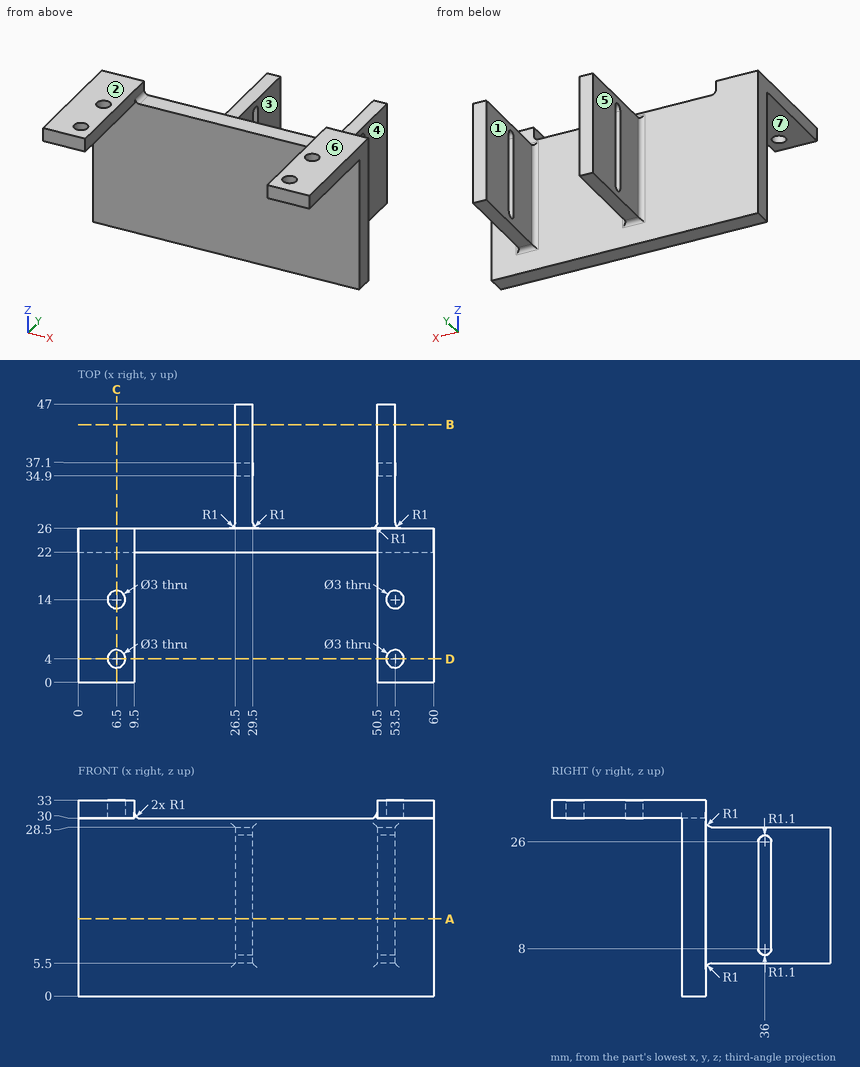
Geometry check sheet. Reference: drawing and pictorial views, mm from the part's lowest x, y, z. A direction names the side the tool comes from. Coordinates: 2 decimals unless noted, no trailing zeros. Order: outer loops, then holes, each group sorted by start corner. A loop starts at its lowest first (then second) coordinate and runs counter-clockwise, first axis right, second up. Notation, with made-up numbers: M 7.5,33 L 40.5,33 A19 cw 40.5,51 Z; hole C 56.5,84 d1. An arc over 180 degrees is marked long. Write each question's results on one line, items separated by ' | '. Start each with the question number.
1. Cross-section at A-A on z = 13. Record the cut outline in (x, y), and give its area (3 significant figures).
2. Cross-section at B-B on y = 43.5. Record the cut outline in (x, z).
3. Mould release check, pull along X, two halves, no side actions. Record for the marked faces 1, 2, 3 and 4: +X half, -X half, draft (parallel to the pull), parting line (faces both ways), or undercut.
4. Cross-section at C-C on x = 6.5. Record the cut outline in (y, z), and give its area (3 significant figures).
5. Access from +Z, -Z, +X, -X, +Y, -Y to the whole of each face (thin tool, end or side, straight path). Record for the marked faces 5, 6 and 7.
6. Cross-section at D-D on y = 4. Record the cut outline in (x, z), and give its area (3 significant figures).
7. Material ranges on probe 1 along Y at (x, z) = (53.5, 32.15); probe 2 along X at (y, z) = (45, 23); probe 3 along X at (y, z) = (19, 31), recorded low to high.
8. Go/stop test with flat-tipped pins: P1, Ø1.8, axis at x = 53.5, y = 4, coming from the +Z side; P2, Ø4, axis at x = 6.5, y = 14, coming from the -Z side; P3, Ø2, axis at x = 13, y = 23, coming from the +Z side; P4, Ø2.5, axis at x = 51.5, z = 16, coming from the -Y side. Record where each tip stops, or that it passes through.
Checks:
1) outline: M 0,22 L 60,22 L 60,26 L 54.5,26 A1 cw 53.5,27 L 53.5,34.9 L 50.5,34.9 L 50.5,27 A1 cw 49.5,26 L 30.5,26 A1 cw 29.5,27 L 29.5,34.9 L 26.5,34.9 L 26.5,27 A1 cw 25.5,26 L 0,26 Z; M 26.5,37.1 L 29.5,37.1 L 29.5,47 L 26.5,47 Z; M 50.5,37.1 L 53.5,37.1 L 53.5,47 L 50.5,47 Z | area: 354 mm²
2) outline: M 26.5,5.5 L 29.5,5.5 L 29.5,28.5 L 26.5,28.5 Z; M 50.5,5.5 L 53.5,5.5 L 53.5,28.5 L 50.5,28.5 Z
3) face 1: undercut | face 2: draft | face 3: undercut | face 4: +X half
4) outline: M 0,30 L 2.5,30 L 2.5,33 L 0,33 Z; M 5.5,30 L 12.5,30 L 12.5,33 L 5.5,33 Z; M 15.5,30 L 22,30 L 22,0 L 26,0 L 26,33 L 15.5,33 Z | area: 180 mm²
5) face 5: +Z, -Z, -X, +Y | face 6: +Z, +X, -X, +Y, -Y | face 7: -Z, +X, -X, -Y
6) outline: M 0,30 L 5,30 L 5,33 L 0,33 Z; M 8,30 L 9.5,30 L 9.5,33 L 8,33 Z; M 50.5,30 L 52,30 L 52,33 L 50.5,33 Z; M 55,30 L 60,30 L 60,33 L 55,33 Z | area: 39.0 mm²
7) probe 1: y = 0 to 2.5, 5.5 to 12.5, 15.5 to 26 | probe 2: x = 26.5 to 29.5, 50.5 to 53.5 | probe 3: x = 0 to 9.5, 50.5 to 60
8) P1: passes through | P2: stops at z = 30 | P3: stops at z = 30 | P4: stops at y = 22
